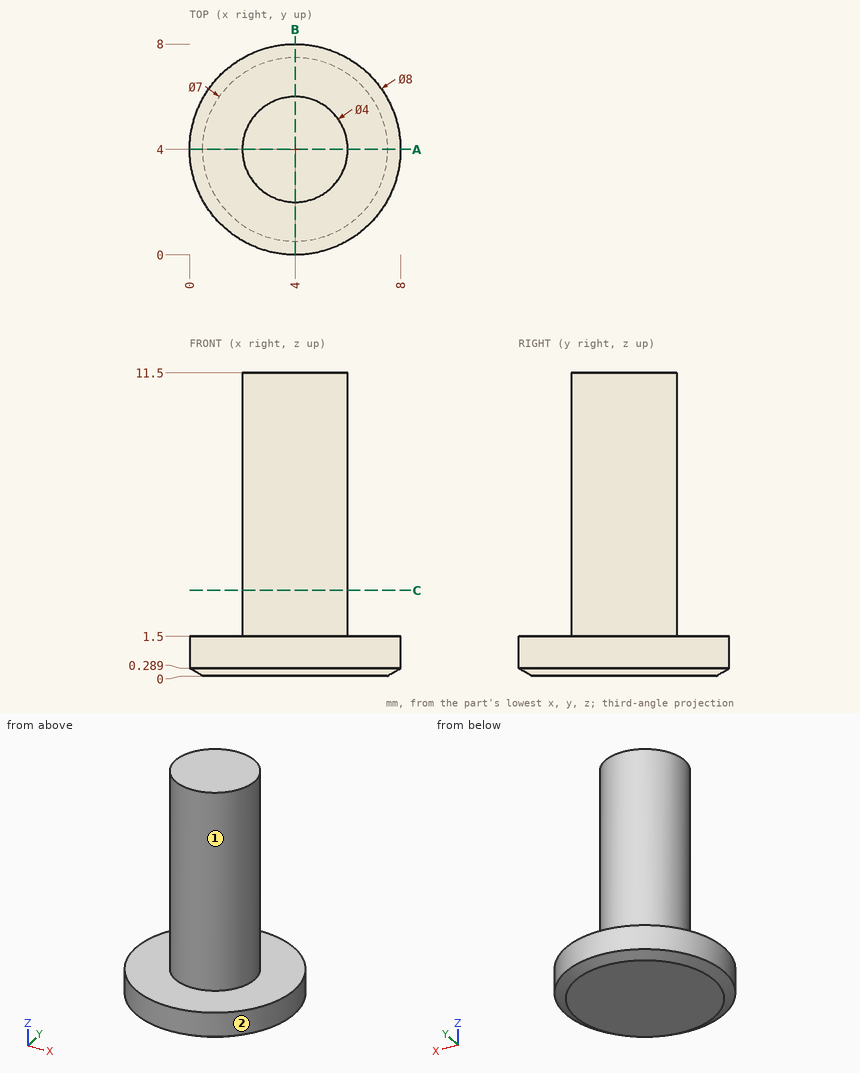
Verification items for this drawing (mm, ordinates from the low corner). A direction names the side the tool comes from. Give positions to 0.01 mm unless a question says otherwise; leave off trailing zeros. Write each loop counter-clockwise with the first axis right and the second up, starting at its lowest first coordinate (ties: lowest second). Pieces come first, ordered by that corner, then holes. Notation, with made-up numbers: (35, 14.5) - (59, 14.5) arc R14 cw to (59, 34.5) - close; hole circle Ø4 at (80, 15.5). An arc over 180 degrees is marked (long way). Answer as a JSON object with one key per item and string values. Group by question number.
1) Thickness scan on probe 1 along Z at (x, y) = (6.5, 3.5); probe 2 along Z at (x, y) = (3, 7.5); probe 3 along Y at (x, z) = (5.5, 8) (1 decimal). Record the ranges inside material, lowest first. Write a range as from..to.
2) Sectioned sample at C-C (z = 3.25). Record the cut outline in (x, y), then the cut area to 3 significant figures.
3) Depth check by flat-ended pin: P1, Ø3, axis at x = 3.5, z = 8, coming from the -Y side; P2, Ø1, axis at y = 2.5, z = 8, coming from the +X side; P3, Ø4, axis at y = 1.5, z = 8.5, coming from the -X side. Enter the tip coordinate at first touch or a pass-through.
4) Access from +Z, -Z, +X, -X, +Y, -Y to the whole of each face (thin tool, end or side, straight path). Record for the marked faces 1 and 2.
5) Sectioned sample at A-A (y = 4). Record the cut outline in (x, z).
Geometry results:
{
 "1": {"probe 1": "z = 0..1.5", "probe 2": "z = 0.08..1.5", "probe 3": "y = 2.7..5.3"},
 "2": {"outline": "circle Ø4 at (4, 4)", "area": "12.6 mm^2"},
 "3": {"P1": "stops at y = 2", "P2": "stops at x = 5.73", "P3": "stops at x = 2.06"},
 "4": {"face 1": "+Z", "face 2": "+Z, -Z"},
 "5": {"outline": "(0, 0.29) - (0.5, 0) - (7.5, 0) - (8, 0.29) - (8, 1.5) - (6, 1.5) - (6, 11.5) - (2, 11.5) - (2, 1.5) - (0, 1.5) - close"}
}
